Drawing for the job (mm, zero at the part's lowest x, y, z). A direction names the side the tool comes from. Give positions to 0.01 mm unless a question says otherwise; leave off trailing zeros. Order: outer loops, then holes, each group sorted by start corner. A loop starts at its lowest first (then second) coordinate and runs counter-clockwise, first axis right, second up. Notation, with made-up numbers: (81.5, 27) - (128.5, 27) arc R25 cw to (128.5, 41) - close; hole circle Ø8 at (45.25, -34.75). An arc over 180 degrees is marked (long way). Use CSV: the item, a comma, the result in double quotes. Start each with the question number.
(1) Band-saw the part on A-A, the plane y = 18.75. Give the cut face in (x, z).
(2) Tool access for the marked faces 5 and 6: list every direction of +Z, -Z, +X, -X, +Y, -Y with a clear straight run to the whole face (end or side of a thin tool).
(3) Band-saw the part on B-B, the plane y = 10.75. Give the cut face in (x, z).
(4) Pull direction X, two halves, no side cores. Call the marked faces 1, 2, 3 and 4: +X half, -X half, draft (parallel to the pull), parting line (faces both ways), or undercut.
(5) Drop flat-ended pins along their axis: pin 1 Ø10 at (y, z) = (9.5, 3) entering from +X; pin 2 Ø2 at (y, z) = (7.5, 17.5) entering from +X; pin 3 Ø4 at (x, z) = (8, 22) entering from -Y; pin 4 Ø6 at (x, z) = (8.5, 7) entering from -Y. Give the stop position or say it passes through.
(6) Probe L1, parallel to Y at x = 3.75, z = 17.75; L2, parallel to Y at x = 10.5, z = 16.5; L3, parallel to X at y = 14.75, z = 16.5. List the from-to ranges inside material, lowest first.
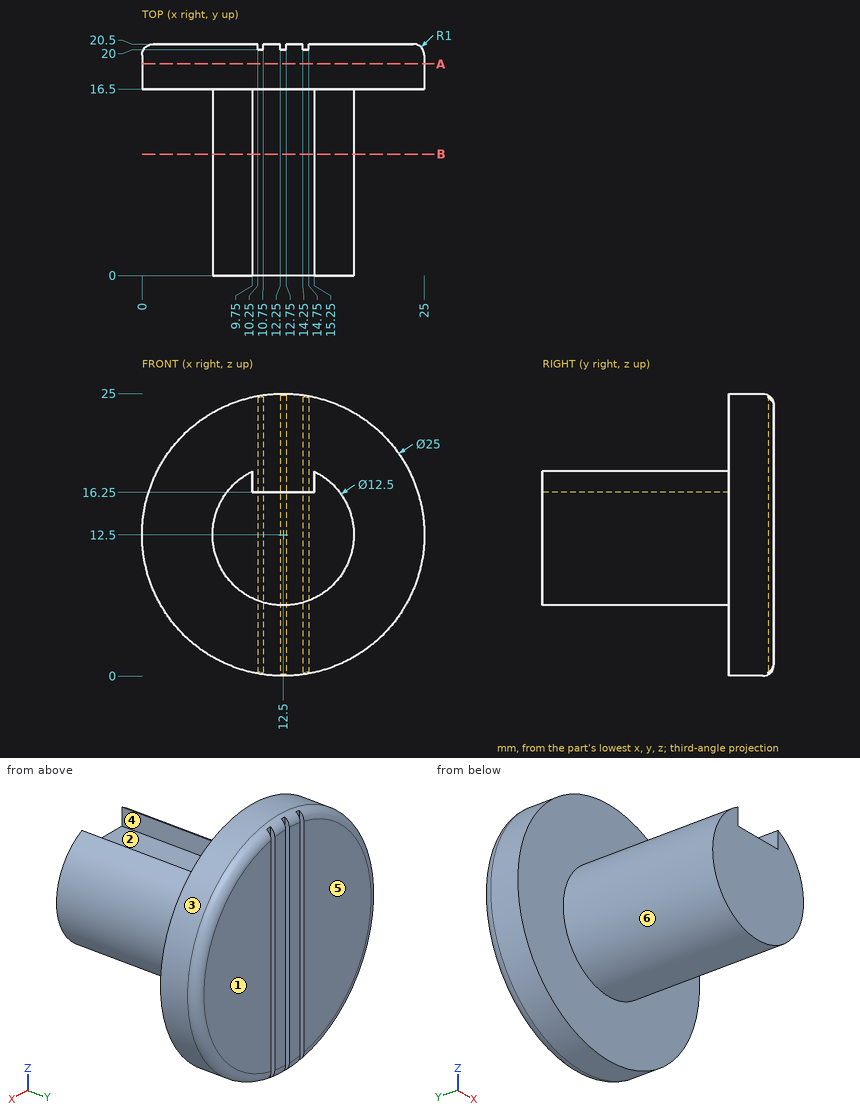
Answer block:
1,outline,"circle Ø25 at (12.5, 12.5)"
2,face 5,"+Z, -Z, +X, -X, +Y"
2,face 6,"-Y"
3,outline,"(9.75, 16.25) - (9.75, 18.11) arc R6.25 ccw (long way) to (15.25, 18.11) - (15.25, 16.25) - close"
4,face 1,"draft"
4,face 2,"undercut"
4,face 3,"parting line"
4,face 4,"undercut"
5,pin 1,"stops at x = 16.84"
5,pin 2,"stops at x = 17.3"
5,pin 3,"stops at y = 16.5"
5,pin 4,"stops at y = 0"
6,L1,"y = 16.5 to 20.5"
6,L2,"y = 16.5 to 20"
6,L3,"x = 7.7 to 9.75, 15.25 to 17.3"
